The listing builds one solid part. Answer for the finished solid, in the listing's coordinates (mm). Face numbers are marked on the shaded views. A direction names the side the tool comes from. Round coordinates to 2 decimals unless told otherwise and drop trailing zeros. Write each loop counter-clockwise with the first axis right and the second up, starting at its lowest first coordinate (ties: lowest second). Pieces come first, ordered by that corner, then holes. Notation, with made-up numbers: (17, 9) -> (66, 9) arc R21 ccw to (66, 42) -> close; hole circle Ø3 at (43, 54.25). An arc over 180 degrees is marked (long way). Write each question's results on one line, items separated by ' | '. Start each with the question number.
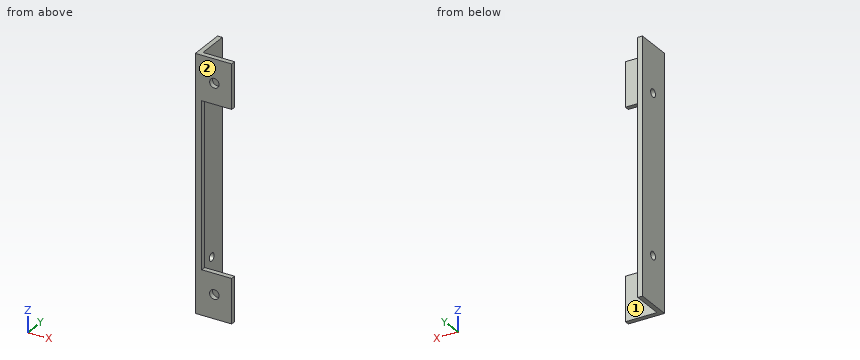
```python
from build123d import *

# Parameters (mm, degrees)
EXTRU_MINCE1_DEPTH      = 80
ESQUISSE2_R             = 1.25
ENL_V_MAT_EXTRU_1_DEPTH = 10
ESQUISSE3_R             = 1.5
ESQUISSE3_W             = 9.5
ESQUISSE3_H             = 52
ENL_V_MAT_EXTRU_2_DEPTH = 10


with BuildPart() as part:
    # Esquisse1 → Extru.-Mince1 (new body)
    with BuildSketch(Plane.XY):
        Polygon((0, 11.5), (0, 0), (11.5, 0), (11.5, 1.5), (1.5, 1.5), (1.5, 11.5), align=None)
    extrude(amount=EXTRU_MINCE1_DEPTH)

    # Esquisse2 → Enlèv. mat.-Extru.1 (cut)
    with BuildSketch(Plane.ZY):
        with Locations(Location((15, 6, 0), (0, 0, 270))):
            Circle(ESQUISSE2_R)
        with Locations(Location((65, 6, 0), (0, 0, 90))):
            Circle(ESQUISSE2_R)
    extrude(amount=-ENL_V_MAT_EXTRU_1_DEPTH, mode=Mode.SUBTRACT)

    # Esquisse3 → Enlèv. mat.-Extru.2 (cut)
    with BuildSketch(Plane.XZ):
        with Locations(Location((6, 7.5, 0), (0, 0, 270))):
            Circle(ESQUISSE3_R)
        with Locations(Location((6, 72.5, 0), (0, 0, 90))):
            Circle(ESQUISSE3_R)
        with Locations((6.75, 40)):
            Rectangle(ESQUISSE3_W, ESQUISSE3_H)
    extrude(amount=-ENL_V_MAT_EXTRU_2_DEPTH, mode=Mode.SUBTRACT)


solid = part.part
```
Q1. The part is cut by section C-C, the plane z = 72.5. Write down the section's boundary in (x, y), then the cut area to 4 significant figures.
Q2. The part is cut by section A-A, the plane x = 9.25. Write down the section's boundary in (y, z), then the cut area to 3 significant figures.
Q3. For the marked faces 1 and 2, determine the directions among +Z, -Z, +X, -X, +Y, -Y from which every point of the face is accessible in a straight line to the end or side of a thin tool.
Q4. Each of these flat-tipped pins is pushed along its axis until it touches: pin 1 (4 mm diameter, centred on x = 2.5, y = 9.5, fed in from +Z); pin 2 (4 mm diameter, centred on y = 6, z = 65, fed in from +X); pin 3 (1.6 mm diameter, centred on y = 0.5, z = 32.5, fed in from +X). Where does it stop, or does it pass through?
Q5. The part is cut by section B-B, the plane y = 6. Write down the section's boundary in (x, z), then the cut area to 4 significant figures.
Q6. The part is cut by section D-D, the plane x = 6. Write down the section's boundary in (y, z), then the cut area to 3 significant figures.
Q7. Find the intervals of material crossed by line 1 (Z direction, x = 0.85, y = 6); line 2 (Y direction, x = 0.85, z = 65); line 3 (X direction, y = 8.75, z = 3.5), in increasing order.
Answers follow:
1) outline: (0, 0) -> (4.5, 0) -> (4.5, 1.5) -> (1.5, 1.5) -> (1.5, 11.5) -> (0, 11.5) -> close; (7.5, 0) -> (11.5, 0) -> (11.5, 1.5) -> (7.5, 1.5) -> close | area: 27.75 mm^2
2) outline: (0, 0) -> (1.5, 0) -> (1.5, 14) -> (0, 14) -> close; (0, 66) -> (1.5, 66) -> (1.5, 80) -> (0, 80) -> close | area: 42.0 mm^2
3) face 1: +Z, -Z, +X, +Y | face 2: +Z, -Z, +X, -X, -Y
4) pin 1: z = 80 | pin 2: x = 1.5 | pin 3: x = 2
5) outline: (0, 0) -> (1.5, 0) -> (1.5, 13.75) -> (0, 13.75) -> close; (0, 16.25) -> (1.5, 16.25) -> (1.5, 63.75) -> (0, 63.75) -> close; (0, 66.25) -> (1.5, 66.25) -> (1.5, 80) -> (0, 80) -> close | area: 112.5 mm^2
6) outline: (0, 0) -> (1.5, 0) -> (1.5, 6) -> (0, 6) -> close; (0, 9) -> (1.5, 9) -> (1.5, 14) -> (0, 14) -> close; (0, 66) -> (1.5, 66) -> (1.5, 71) -> (0, 71) -> close; (0, 74) -> (1.5, 74) -> (1.5, 80) -> (0, 80) -> close | area: 33.0 mm^2
7) line 1: 0 to 13.75, 16.25 to 63.75, 66.25 to 80 | line 2: 0 to 4.75, 7.25 to 11.5 | line 3: 0 to 1.5
